Part print with two shaded views. Sizes in mm from the minimum x, y, z corner. Round coordinates to 2 decimals unless told otherwise and drop trailing zeros. Return JSON: item names as keys, results as strings. Group by question number.
(1) Drop flat-ended pins along their axis: pin 1 Ø1 at (x, z) = (80, 21.5) entering from -Y; pin 2 Ø1.5 at (y, z) = (34.5, 4) entering from +X. Give the stop position or say it passes through.
(2) Mould opens along Y. For the marked faces 1, 2 and 3 say: +Y half, -Y half, draft (parallel to the pull), parting line (faces both ways), or undercut.
(3) Drill centre lines: L1, parallel to X at y = 11.5, z = 35; L2, parallel to X at y = 19.5, z = 38.5. Where is each one in solid material? Low to high. Write a range as from..to.
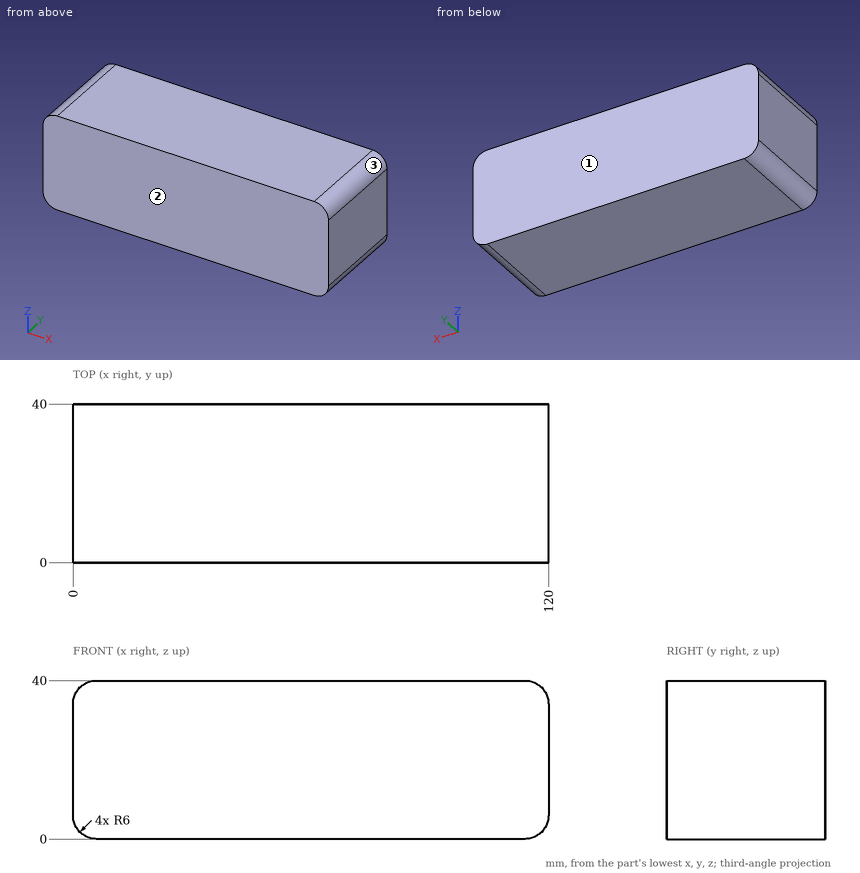
Computed values:
{
 "1": {"pin 1": "y = 0", "pin 2": "x = 119.87"},
 "2": {"face 1": "+Y half", "face 2": "-Y half", "face 3": "draft"},
 "3": {"L1": "0.08..119.92", "L2": "2.03..117.97"}
}
